Verification items for this drawing (mm, ordinates from the low corner). A direction names the side the tool comes from. Coordinates: 2 decimals unless noted, no trailing zeros. Order: outer loops, then holes, each group sorted by start corner. A loop starts at its lowest first (then second) coordinate and runs counter-clockwise, first axis right, second up. Notation, with made-up numbers: (48, 7) -> (81, 7) arc R33 cw to (81, 37) -> close; hole circle Ø4 at (54, -36.5). An arc over 180 degrees is marked (long way). Write item = value, one per line. Start each with the question number.
1. Release check for a two-part mould opening along X. For the marked faces 1, 2, 3 and 4 record: +X half, -X half, draft (parallel to the pull), parting line (faces both ways), or undercut.
2. Thickness scan on line 1 along X through (y, z) = (8.75, 4); line 2 along Y through (x, z) = (7.5, 4.75); line 3 along X through (y, z) = (4, 6.25). Record the ranges inside material, lowest first. Write a range as from..to.
3. Cross-section at D-D on x = 5. Record the cut outline in (y, z).
4. Cross-section at B-B on y = 8.75. Record the cut outline in (x, z).
5. Cross-section at A-A on y = 5.5. Record the cut outline in (x, z), plus the area to 3 significant figures.
6. Cross-section at C-C on x = 17. Record the cut outline in (y, z), plus the area to 3 significant figures.
7. Set-up check for the marked faces 5, 6 and 7: record each of +Z, -Z, +X, -X, +Y, -Y from which the full face is reachable in a straight line by a thin tool's end or side.
8. Go/stop test with flat-tipped pins: P1, Ø2.5, axis at x = 20, z = 4, coming from the +Y side; P2, Ø1.8, axis at y = 3.5, z = 4.5, coming from the -X side; P3, Ø1, axis at y = 6.5, z = 2.5, coming from the +X side. Record where each tip stops, or that it passes through.
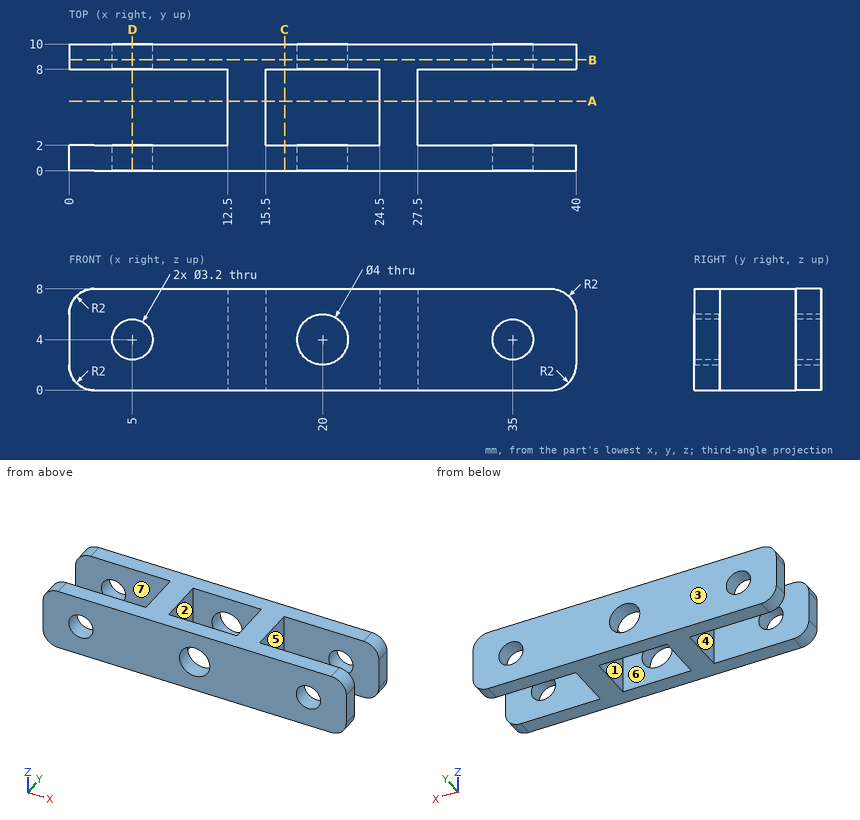
Worked out:
q1.face_1 = undercut
q1.face_2 = undercut
q1.face_3 = draft
q1.face_4 = -X half
q2.line_1 = 0..3.4, 6.6..18, 22..33.4, 36.6..40
q2.line_2 = 0..2, 8..10
q2.line_3 = 12.5..15.5, 24.5..27.5
q3.outline = (0, 0) -> (2, 0) -> (2, 2.4) -> (0, 2.4) -> close; (0, 5.6) -> (2, 5.6) -> (2, 8) -> (0, 8) -> close; (8, 0) -> (10, 0) -> (10, 2.4) -> (8, 2.4) -> close; (8, 5.6) -> (10, 5.6) -> (10, 8) -> (8, 8) -> close
q4.outline = (0, 2) arc R2 ccw to (2, 0) -> (38, 0) arc R2 ccw to (40, 2) -> (40, 6) arc R2 ccw to (38, 8) -> (2, 8) arc R2 ccw to (0, 6) -> close; hole circle Ø3.2 at (5, 4); hole circle Ø4 at (20, 4); hole circle Ø3.2 at (35, 4)
q5.outline = (12.5, 0) -> (15.5, 0) -> (15.5, 8) -> (12.5, 8) -> close; (24.5, 0) -> (27.5, 0) -> (27.5, 8) -> (24.5, 8) -> close
q5.area = 48.0 mm²
q6.outline = (0, 0) -> (2, 0) -> (2, 8) -> (0, 8) -> close; (8, 0) -> (10, 0) -> (10, 8) -> (8, 8) -> close
q6.area = 32.0 mm²
q7.face_5 = +Z, -Z, +X
q7.face_6 = +Z, -Z
q7.face_7 = +Z, -Z, -X
q8.P1 = through
q8.P2 = 12.5
q8.P3 = 27.5
